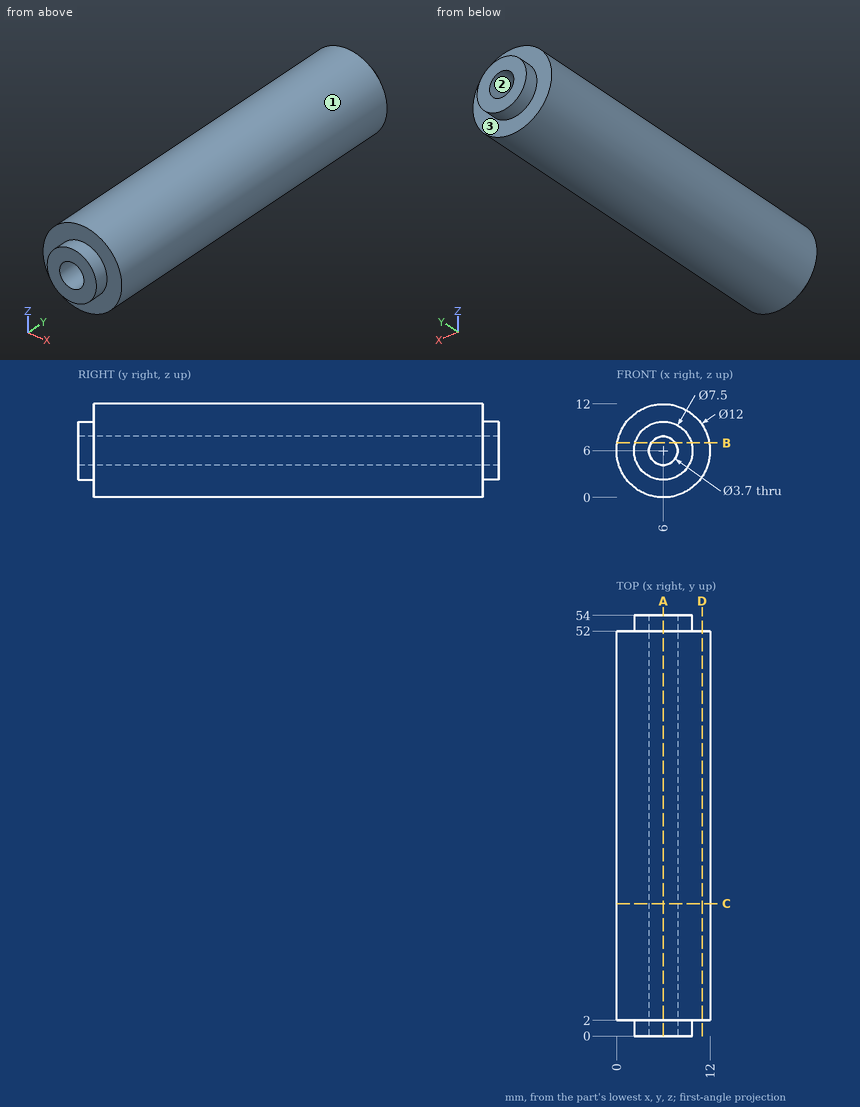
Check sheet for the drawn part. Datum: minimum x, y, z corner. Units: mm. Round coordinates to 2 decimals unless told otherwise and drop trailing zeros. Order: outer loops, then holes, each group sorted by start corner. A loop starts at its lowest first (then second) coordinate and runs counter-clockwise, first axis right, second up.
(1) Cross-section at A-A, the plane x = 6. Enter the section's corners in (y, z).
(2) Cross-section at C-C, the plane y = 17. Enter the section's corners in (x, z), and give its area (3 significant figures).
(3) Cross-section at B-B, the plane z = 7. Enter the section's corners in (x, y).
(4) Go/stop test with flat-tipped pins: P1, Ø5, axis at x = 9.5, y = 34, coming from the +Z side; P2, Ø1, axis at x = 10, y = 16, coming from the +Z side; P3, Ø3, axis at x = 6, z = 6, coming from the -Y side (1 decimal); P4, Ø5, axis at y = 44, z = 1.5, coming from the +X side. Record where each tip stops, or that it passes through.
(5) Scan lines: probe 1 along Z at (x, y) = (6, 43.5); probe 2 along Y at (x, z) = (10.75, 3.5); probe 3 along X at (y, z) = (31.5, 5.25). Record each from-to range of solid material in increasing order.
(6) Cross-section at D-D, the plane x = 11. Enter the section's corners in (y, z).
(7) Draft check along Z on the marked faces 1, 2 and 3. Enter one of: pulls with the +Z half, pulls with the -Z half, needs draft (parallel to the pull), parting line crosses it, or undercut.
Check sheet entries:
1. outline: (0, 2.25) - (2, 2.25) - (2, 0) - (52, 0) - (52, 2.25) - (54, 2.25) - (54, 4.15) - (0, 4.15) - close; (0, 7.85) - (54, 7.85) - (54, 9.75) - (52, 9.75) - (52, 12) - (2, 12) - (2, 9.75) - (0, 9.75) - close
2. outline: circle Ø12 at (6, 6); hole circle Ø3.7 at (6, 6)
2. area: 102 mm2
3. outline: (0.08, 2) - (2.39, 2) - (2.39, 0) - (4.44, 0) - (4.44, 54) - (2.39, 54) - (2.39, 52) - (0.08, 52) - close; (7.56, 0) - (9.61, 0) - (9.61, 2) - (11.92, 2) - (11.92, 52) - (9.61, 52) - (9.61, 54) - (7.56, 54) - close
4. P1: stops at z = 11.92
4. P2: stops at z = 10.87
4. P3: passes through
4. P4: stops at x = 11.66
5. probe 1: z = 0 to 4.15, 7.85 to 12
5. probe 2: y = 2 to 52
5. probe 3: x = 0.05 to 4.31, 7.69 to 11.95
6. outline: (2, 2.68) - (52, 2.68) - (52, 9.32) - (2, 9.32) - close
7. face 1: parting line crosses it
7. face 2: undercut
7. face 3: needs draft
